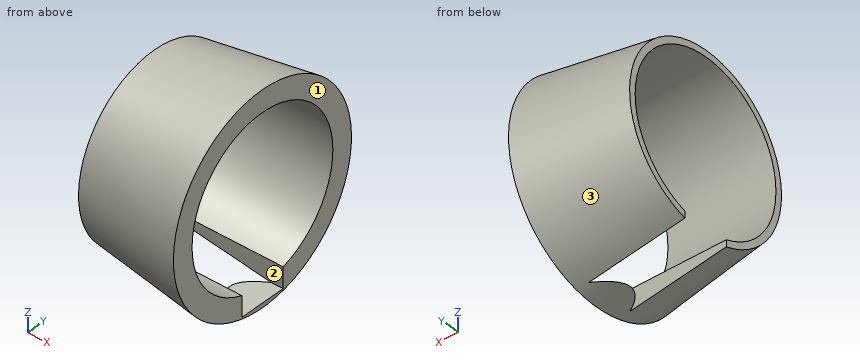
```python
from build123d import *

# Parameters (mm, degrees)
F2_W     = 20
F2_H     = 16.608118
F3_DEPTH = 45.001


with BuildPart() as f1:
    # F0 (on Front) → F1 (revolve)
    with BuildSketch(Plane.XZ):
        Polygon((-22.5, 36.675662), (-22.5, 34), (22.5, 34), (22.5, 43), align=None)
    revolve(axis=Axis((3.817478, 0, 0), (1, 0, 0)))

    # F2 (on face) → F3 (cut, through all)
    with BuildSketch(Plane.YZ.offset(22.5)):
        with Locations((0, -32.795941)):
            Rectangle(F2_W, F2_H)
    extrude(amount=-F3_DEPTH, mode=Mode.SUBTRACT)


solid = f1.part
```
Geometry check sheet. Reference: the model listing, model coordinates, mm. Face numbers are marked on the shaded views. Coordinates: 2 decimals unless noted, no trailing zeros. Loops run counter-clockwise (first coordinate to the right, second up) from the corner with the lowest first, then second, coordinate; pieces in that order, holes last.
Item 1: Go/stop test with flat-tipped pins: pin 1 Ø10 at (x, y) = (-13.5, 15.5) entering from -Z; pin 2 Ø8 at (x, y) = (9.5, -0.5) entering from -Z; pin 3 Ø10 at (x, z) = (-4, -21.5) entering from +Y. Record where each tip stops, or that it passes through.
Item 2: Release check for a two-part mould opening along Z. For the marked faces 1, 2 and 3 record: released by +Z, released by -Z, zero draft, split by the parting line, or undercut.
Item 3: Thickness scan on line 1 (Y direction, x = 1, z = 16); line 2 (Y direction, x = 7.5, z = 30); line 3 (Z direction, x = 9.5, y = 30.5). Record the ranges inside material, lowest first.
Item 4: Sectioned sample at B-B, the plane x = -10.5. Record the boundary of the cut face in (y, z), then the cut area to 3 significant figures.
Item 5: Sectioned sample at A-A, the plane z = 0. Record the boundary of the cut face in (x, y).
Check result:
1. pin 1: stops at z = -36.63
1. pin 2: stops at z = -41.73
1. pin 3: stops at y = 35.77
2. face 1: zero draft
2. face 2: undercut
2. face 3: split by the parting line
3. line 1: y = -36.64 to -30, 30 to 36.64
3. line 2: y = -27.79 to -16, 16 to 27.79
3. line 3: z = -27.66 to -15.02, 15.02 to 27.66
4. outline: (-10, -37.04) - (-10, -32.5) arc R34 cw (long way) to (10, -32.5) - (10, -37.04) arc R38.36 ccw (long way) to start
4. area: 903 mm2
5. outline: (-22.5, -36.68) - (22.5, -43) - (22.5, -34) - (-22.5, -34) - close; (-22.5, 34) - (22.5, 34) - (22.5, 43) - (-22.5, 36.68) - close
